Model file for the job. Use its own axes, mm. A direction names the side the tool comes from. Give positions to 0.01 mm unless a question says otherwise; leave off trailing zeros. Loops run counter-clockwise (first coordinate to the right, second up) from the corner with the lowest first, then second, coordinate; pieces in that order, holes last. Notation, with made-up numbers: M -26.5,-5.5 L 0.5,-5.5 A7 cw 0.5,1.5 Z; hole C -21.75,-31 d7. An arc over 180 degrees is marked long. Answer in a Markdown table with one row per item.
```python
from build123d import *
from build123d.topology import SkipClean

# Parameters (mm, degrees)
SKETCH1_R                = 4.1
SKETCH1_R_2              = 4
SKETCH1_R_3              = 2.6
BOSS_EXTRUDE1_DEPTH      = 10
CUT_EXTRUDE1_START       = -4
CUT_EXTRUDE1_DEPTH       = 4
BOSS_EXTRUDE2_DEPTH      = 10
BOSS_EXTRUDE2_DEPTH_BACK = 10
SKETCH5_R                = 4
FILLET1_R                = 1
BOSS_EXTRUDE3_START      = 10
SKETCH6_R                = 2.6
BOSS_EXTRUDE3_DEPTH      = 10
BOSS_EXTRUDE4_DEPTH      = 20
CUT_EXTRUDE2_REACH       = 125.31
FILLET2_R                = 10
FILLET3_R                = 2


with BuildPart() as part:
    # Sketch1 → Boss-Extrude1 (new body)
    with BuildSketch(Plane(origin=(0, 0, 0), x_dir=(1, 0, 0), z_dir=(0, 1, 0))):
        with BuildLine():
            Line((28.853428594, -0.793287448), (1.853428594, -0.793287448))
            ThreePointArc((1.853428594, -0.793287448), (-1.682105312, 0.671178646), (-3.146571406, 4.206712552))
            Line((-3.146571406, 4.206712552), (-3.146571406, 6.206712552))
            ThreePointArc((-3.146571406, 6.206712552), (-5.489717157, 11.863566801), (-11.146571406, 14.206712552))
            Line((-11.146571406, 14.206712552), (-15.146571406, 14.206712552))
            ThreePointArc((-15.146571406, 14.206712552), (-20.803425656, 11.863566801), (-23.146571406, 6.206712552))
            Line((-23.146571406, 6.206712552), (-23.146571406, -92.793287448))
            ThreePointArc((-23.146571406, -92.793287448), (-24.025251062, -94.914607792), (-26.146571406, -95.793287448))
            Line((-26.146571406, -95.793287448), (-40.146571406, -95.793287448))
            ThreePointArc((-40.146571406, -95.793287448), (-42.26789175, -94.914607792), (-43.146571406, -92.793287448))
            Line((-43.146571406, -92.793287448), (-43.146571406, 4.206712552))
            Line((-43.146571406, 4.206712552), (-43.146571406, 26.206712552))
            ThreePointArc((-43.146571406, 26.206712552), (-40.803425656, 31.863566801), (-35.146571406, 34.206712552))
            Line((-35.146571406, 34.206712552), (-3.146571406, 34.206712552))
            Line((-3.146571406, 34.206712552), (25.853428594, 34.206712552))
            ThreePointArc((25.853428594, 34.206712552), (31.510282843, 31.863566801), (33.853428594, 26.206712552))
            Line((33.853428594, 26.206712552), (33.853428594, 4.206712552))
            ThreePointArc((33.853428594, 4.206712552), (32.3889625, 0.671178646), (28.853428594, -0.793287448))
        make_face()
        with Locations(Location((25.853428594, 7.206712552, 0), (0, 0, 270))):
            Circle(SKETCH1_R, mode=Mode.SUBTRACT)
        with Locations(Location((4.853428594, 7.206712552, 0), (0, 0, 270))):
            Circle(SKETCH1_R_2, mode=Mode.SUBTRACT)
        with Locations(Location((-31.146571406, -87.793287448, 0), (0, 0, 270))):
            Circle(SKETCH1_R_3, mode=Mode.SUBTRACT)
        with Locations(Location((-31.146571406, -60.793287448, 0), (0, 0, 270))):
            Circle(SKETCH1_R_3, mode=Mode.SUBTRACT)
    extrude(amount=BOSS_EXTRUDE1_DEPTH)

    # Sketch2 → Cut-Extrude1 (cut)
    with BuildSketch(Plane(origin=(0, 10, 0), x_dir=(1, 0, 0), z_dir=(0, 1, 0)).offset(CUT_EXTRUDE1_START)):
        with BuildLine():
            Line((25.853428594, 14.706712552), (33.853428594, 14.706712552))
            Line((33.853428594, 14.706712552), (33.853428594, 4.206712552))
            ThreePointArc((33.853428594, 4.206712552), (32.3889625, 0.671178646), (28.853428594, -0.793287448))
            Line((28.853428594, -0.793287448), (18.353428594, -0.793287448))
            Line((18.353428594, -0.793287448), (18.353428594, 7.206712552))
            ThreePointArc((18.353428594, 7.206712552), (20.550127735, 12.510013411), (25.853428594, 14.706712552))
        make_face()
    extrude(amount=CUT_EXTRUDE1_DEPTH, mode=Mode.SUBTRACT)

    # Sketch5 → Boss-Extrude2 (add, two sides: drawn at the far end of the back side and taken through both)
    with BuildSketch(Plane(origin=(0, 0, 0), x_dir=(-1, 0, 0), z_dir=(0, -1, 0)).offset(-BOSS_EXTRUDE2_DEPTH_BACK)):
        with Locations(Location((-4.853428594, 7.206712552, 0), (0, 0, 90))):
            Circle(SKETCH5_R)
    extrude(amount=BOSS_EXTRUDE2_DEPTH + BOSS_EXTRUDE2_DEPTH_BACK)

    # Fillet1
    fillet1_edges = [part.edges().sort_by_distance(p)[0] for p in [
        (4.853428594, 0, -3.206712552),
        (4.853428594, -10, -3.206712552),
    ]]
    fillet(fillet1_edges, radius=FILLET1_R)

    # Sketch6 → Boss-Extrude3 (add)
    with SkipClean():  # the faces are left unmerged after this step: merging them gives an invalid solid
        with BuildSketch(Plane.XZ.offset(BOSS_EXTRUDE3_START)):
            with BuildLine():
                Line((-26.146571406, 95.793287448), (-40.146571406, 95.793287448))
                ThreePointArc((-40.146571406, 95.793287448), (-42.26789175, 94.914607792), (-43.146571406, 92.793287448))
                Line((-43.146571406, 92.793287448), (-43.146571406, 51.031484515))
                Line((-43.146571406, 51.031484515), (-23.146571406, 51.031484515))
                Line((-23.146571406, 51.031484515), (-23.146571406, 92.793287448))
                ThreePointArc((-23.146571406, 92.793287448), (-24.025251062, 94.914607792), (-26.146571406, 95.793287448))
            make_face()
            with Locations(Location((-31.146571406, 87.793287448, 0), (0, 0, 270))):
                Circle(SKETCH6_R, mode=Mode.SUBTRACT)
            with Locations(Location((-31.146571406, 60.793287448, 0), (0, 0, 270))):
                Circle(SKETCH6_R, mode=Mode.SUBTRACT)
        extrude(amount=-BOSS_EXTRUDE3_DEPTH)

    # Sketch7 → Boss-Extrude4 (add)
    with SkipClean():  # the faces are left unmerged after this step: merging them gives an invalid solid
        with BuildSketch(Plane(origin=(-23.146571406, 0, 0), x_dir=(0, 0, -1), z_dir=(1, 0, 0))):
            Polygon((-51.031484515, -10), (-45.232749266, 0), (-51.031484515, 0), align=None)
        extrude(amount=-BOSS_EXTRUDE4_DEPTH)

    # Cut-Extrude2: up to this face of the body (flat: up to its plane)
    cut_extrude2_end = Plane(part.part.faces().sort_by_distance((-23.146571406, 5, 43.293287448))[0])
    # Sketch8 → Cut-Extrude2 (cut, up to the picked face)
    with BuildSketch(Plane.ZY.offset(43.146571406), mode=Mode.PRIVATE) as cut_extrude2_sk1:
        Polygon((53.911938049, -5), (48.1132028, 5), (-1.206712552, 10), (103.677305794, 10), (103.677305794, -5), align=None)
    cut_extrude2_tool1 = split(extrude(cut_extrude2_sk1.sketch, amount=-CUT_EXTRUDE2_REACH, mode=Mode.PRIVATE), bisect_by=cut_extrude2_end, keep=Keep.BOTH, mode=Mode.PRIVATE)
    add(cut_extrude2_tool1.solids().sort_by(Axis((-43.146571, 3.405459, 70.825985), (1, 0, 0)))[0], mode=Mode.SUBTRACT)

    # Fillet2
    fillet2_edges = [part.edges().sort_by_distance(p)[0] for p in [
        (-33.146571406, 0, 45.232749266),
        (-33.146571406, 5, 48.1132028),
    ]]
    fillet(fillet2_edges, radius=FILLET2_R)

    # Fillet3
    fillet3_edges = [part.edges().sort_by_distance(p)[0] for p in [
        (-33.146571406, -10, 51.031484515),
        (-33.146571406, -5, 53.911938049),
    ]]
    fillet(fillet3_edges, radius=FILLET3_R)


solid = part.part
```
Q1. Drop flat-ended pins along their axis: pin 1 (3 mm diameter, centred on x = 21.5, y = 2.5, fed in from +Z); pin 2 (4.5 mm diameter, centred on x = -12.5, y = 6.5, fed in from +Z); pin 3 (1.5 mm diameter, centred on y = -6, z = -9, fed in from -X). Give the stop position or say it passes through.
Reported:
| item | result |
|---|---|
| pin 1 | z = 0.79 |
| pin 2 | z = -14.16 |
| pin 3 | x = 0.99 |
Q2. Probe probe 1 along X at (y, z) = (0.25, -4.5); probe 2 along Y at (x, z) = (-37, 73); probe 3 along X at (y, z) = (5.75, 15.5). List the from-to ranges inside material, lowest first.
Reported:
| item | result |
|---|---|
| probe 1 | -43.15 to -23.15, -3.15 to 22.77, 28.93 to 33.85 |
| probe 2 | -10 to -5 |
| probe 3 | -43.15 to -23.15 |
Q3. Saw through at B-B (x = 16). Give the cut face in (y, z), and give its area (3 significant figures).
Reported:
| item | result |
|---|---|
| outline | M 0,-34.21 L 10,-34.21 L 10,0.79 L 0,0.79 Z |
| area | 350 mm² |
Q4. 3-axis set-ups, long thin cutter, end or side, ignore diameter. For faces 1 (the face through (-33, -5, 76)), 2 (the face through (20.49, 7.97, -12.45)), 3 (the face through (-43.147, 2, 21)), 4 (the face through (-13, 5, -14.207)), 5 (the face through (-5, 5, -34.207)): which of +Z, -Z, +X, -X, +Y, -Y reach the whole face in a straight line?
Reported:
| item | result |
|---|---|
| face 1 | +Z, +X, -X, +Y |
| face 2 | +Z, +X, +Y |
| face 3 | +Z, -Z, -X, +Y, -Y |
| face 4 | +Z, +Y, -Y |
| face 5 | -Z, +X, -X, +Y, -Y |
Q5. Saw through at A-A (y = -7.75). Give the cut face in (x, z), and give its area (3 significant figures).
Reported:
| item | result |
|---|---|
| outline | M -43.15,49.73 L -23.15,49.73 L -23.15,92.79 A3 ccw -26.15,95.79 L -40.15,95.79 A3 ccw -43.15,92.79 Z; C 4.85,-7.21 d8; hole C -31.15,60.79 d5.2; hole C -31.15,87.79 d5.2 |
| area | 925 mm² |
Q6. Saw through at C-C (y = 2). Give the cut face in (x, z).
Reported:
| item | result |
|---|---|
| outline | M -43.15,-26.21 A8 ccw -35.15,-34.21 L 25.85,-34.21 A8 ccw 33.85,-26.21 L 33.85,-4.21 A5 ccw 28.85,0.79 L 1.85,0.79 A5 ccw -3.15,-4.21 L -3.15,-6.21 A8 cw -11.15,-14.21 L -15.15,-14.21 A8 cw -23.15,-6.21 L -23.15,49.68 L -43.15,49.68 Z; hole C 25.85,-7.21 d8.2 |
Q7. Saw through at D-D (z = 77). Give the cut face in (x, y), and give its area (3 significant figures).
Reported:
| item | result |
|---|---|
| outline | M -43.15,-10 L -23.15,-10 L -23.15,-5 L -43.15,-5 Z |
| area | 100 mm² |
Q8. Mould opens along X. For faces 6 (the face through (32.43, 2.96, -0.71)), 7 (the face through (-42.24, -7.54, 94.94)), 8 (the face through (-1.64, 4.93, -0.63)), 9 (the face through (30, 6, -5)) say: released by +X, released by -X, zero draft, split by the parting line, or undercut.
Reported:
| item | result |
|---|---|
| face 6 | released by +X |
| face 7 | released by -X |
| face 8 | undercut |
| face 9 | zero draft |
